The listing builds one solid part. Answer for the finished solid, in the listing's coordinates (mm). A direction names the side the tool comes from. Round coordinates to 2 decimals unless told otherwise and drop trailing zeros. Loops run counter-clockwise (first coordinate to the right, second up) from the corner with the lowest first, then second, coordinate; pieces in that order, holes last. Notation, with made-up numbers: (60.5, 21.25) -> (104.5, 21.25) arc R28 cw to (104.5, 47.25) -> close; hole circle Ø1 at (-18, 37). An arc over 180 degrees is marked (long way). Answer in a Markdown table with one row per item. Add a question column.
```python
from build123d import *

# Parameters (mm, degrees)
BOSS_EXTRUDE1_DEPTH = 1.524
CUT_EXTRUDE1_DEPTH  = 1.524
FILLET1_R           = 0.508
BOSS_EXTRUDE2_DEPTH = 6.223
BOSS_EXTRUDE3_START = -1.524
BOSS_EXTRUDE3_DEPTH = 1.524
CUT_EXTRUDE2_START  = -6.223
CUT_EXTRUDE2_DEPTH  = 6.223
FILLET2_R           = 0.254
SKETCH9_W           = 1.905
SKETCH9_H           = 23.876
CUT_EXTRUDE4_DEPTH  = 51.542276073
FILLET3_R           = 0.254


with BuildPart() as part:
    # Sketch2 → Boss-Extrude1 (new body)
    with BuildSketch(Plane(origin=(0, 0, 0), x_dir=(0, 0, -1), z_dir=(1, 0, 0))):
        with BuildLine():
            Line((-10.16, 10.851579944), (-10.16, 9.756379827))
            ThreePointArc((-10.16, 9.756379827), (-8.902698353, 7.16361824), (-6.088278228, 6.54534691))
            ThreePointArc((-6.088278228, 6.54534691), (-1.097578785, 7.201770952), (3.920718614, 6.808496661))
            ThreePointArc((3.920718614, 6.808496661), (7.044965017, 7.926917254), (7.619757818, 11.195157369))
            ThreePointArc((7.619757818, 11.195157369), (4.593793799, 26.843864795), (6.687175028, 42.644379261))
            ThreePointArc((6.687175028, 42.644379261), (5.465660141, 45.611386582), (2.312998216, 45.014767901))
            ThreePointArc((2.312998216, 45.014767901), (-6.944233805, 29.036045126), (-10.16, 10.851579944))
        make_face()
    extrude(amount=BOSS_EXTRUDE1_DEPTH)

    # Sketch3 → Cut-Extrude1 (cut)
    with BuildSketch(Plane(origin=(1.524, 0, 0), x_dir=(0, 0, -1), z_dir=(1, 0, 0))):
        with BuildLine():
            Line((-7.62, 10.851579944), (-7.62, 9.756379827))
            ThreePointArc((-7.62, 9.756379827), (-7.329853466, 9.15805023), (-6.680371899, 9.015372231))
            ThreePointArc((-6.680371899, 9.015372231), (-1.164335672, 9.74089354), (4.382203558, 9.306221955))
            ThreePointArc((4.382203558, 9.306221955), (5.103183497, 9.564319015), (5.23582799, 10.318528273))
            ThreePointArc((5.23582799, 10.318528273), (2.05490982, 26.768577734), (4.25548932, 43.378207999))
            ThreePointArc((4.25548932, 43.378207999), (-4.558282485, 28.164933022), (-7.62, 10.851579944))
        make_face()
    extrude(amount=-CUT_EXTRUDE1_DEPTH, mode=Mode.SUBTRACT)

    # Fillet1
    fillet1_edges = [part.edges().sort_by_distance(p)[0] for p in [
        (0.762, 43.378207999, -4.25548932),
    ]]
    fillet(fillet1_edges, radius=FILLET1_R)

    # Sketch4 → Boss-Extrude2 (add)
    with BuildSketch(Plane.ZY):
        with BuildLine():
            Line((8.89, 9.756379827), (8.89, 10.851579944))
            ThreePointArc((8.89, 10.851579944), (5.751258145, 28.600489074), (-3.284243768, 44.19648795))
            ThreePointArc((-3.284243768, 44.19648795), (-4.86057473, 44.49479729), (-5.471332174, 43.01129363))
            ThreePointArc((-5.471332174, 43.01129363), (-3.32435181, 26.806221264), (-6.427792904, 10.756842821))
            ThreePointArc((-6.427792904, 10.756842821), (-6.074074257, 8.745618135), (-4.151461086, 8.057359308))
            ThreePointArc((-4.151461086, 8.057359308), (1.130957229, 8.471332246), (6.384325063, 7.78035957))
            ThreePointArc((6.384325063, 7.78035957), (8.116275909, 8.160834235), (8.89, 9.756379827))
        make_face()
        with BuildLine():
            Line((7.62, 9.756379827), (7.62, 10.851579944))
            ThreePointArc((7.62, 10.851579944), (4.96917921, 26.995100943), (-2.704895567, 41.443239142))
            ThreePointArc((-2.704895567, 41.443239142), (-3.329273356, 41.593156599), (-3.601704042, 41.011689155))
            ThreePointArc((-3.601704042, 41.011689155), (-2.10574247, 25.541961828), (-5.23582799, 10.318528273))
            ThreePointArc((-5.23582799, 10.318528273), (-5.103183497, 9.564319015), (-4.382203558, 9.306221955))
            ThreePointArc((-4.382203558, 9.306221955), (1.164335672, 9.74089354), (6.680371899, 9.015372231))
            ThreePointArc((6.680371899, 9.015372231), (7.329853466, 9.15805023), (7.62, 9.756379827))
        make_face(mode=Mode.SUBTRACT)
    extrude(amount=BOSS_EXTRUDE2_DEPTH)

    # Sketch5 → Boss-Extrude3 (add)
    with BuildSketch(Plane(origin=(1.524, 0, 0), x_dir=(0, 0, -1), z_dir=(1, 0, 0)).offset(BOSS_EXTRUDE3_START)):
        with BuildLine():
            Line((7.009110806, 43.67080126), (6.148171078, 49.106560771))
            ThreePointArc((6.148171078, 49.106560771), (3.588810081, 46.474083877), (1.217761815, 43.67080126))
            Line((1.217761815, 43.67080126), (6.534669415, 42.12894069))
            ThreePointArc((6.534669415, 42.12894069), (6.765621389, 42.901799905), (7.009110806, 43.67080126))
        make_face()
    extrude(amount=BOSS_EXTRUDE3_DEPTH)

    # Sketch6 → Cut-Extrude2 (cut)
    with BuildSketch(Plane.ZY.offset(6.223).offset(CUT_EXTRUDE2_START)):
        with BuildLine():
            Line((8.89, 9.756379827), (8.89, 10.851579944))
            ThreePointArc((8.89, 10.851579944), (5.751258145, 28.600489074), (-3.284243768, 44.19648795))
            ThreePointArc((-3.284243768, 44.19648795), (-4.86057473, 44.49479729), (-5.471332174, 43.01129363))
            ThreePointArc((-5.471332174, 43.01129363), (-3.32435181, 26.806221264), (-6.427792904, 10.756842821))
            ThreePointArc((-6.427792904, 10.756842821), (-6.074074257, 8.745618135), (-4.151461086, 8.057359308))
            ThreePointArc((-4.151461086, 8.057359308), (1.130957229, 8.471332246), (6.384325063, 7.78035957))
            ThreePointArc((6.384325063, 7.78035957), (8.116275909, 8.160834235), (8.89, 9.756379827))
        make_face()
        with BuildLine():
            Line((8.8646, 9.756379827), (8.8646, 10.851579944))
            ThreePointArc((8.8646, 10.851579944), (5.727398631, 28.591777953), (-3.303668679, 44.180122351))
            ThreePointArc((-3.303668679, 44.180122351), (-4.848473022, 44.472465504), (-5.447015317, 43.018631917))
            ThreePointArc((-5.447015317, 43.018631917), (-3.29896297, 26.805468394), (-6.403953606, 10.74807653))
            ThreePointArc((-6.403953606, 10.74807653), (-6.054656442, 8.761992152), (-4.156075935, 8.082336561))
            ThreePointArc((-4.156075935, 8.082336561), (1.131624798, 8.496723472), (6.390246, 7.805059824))
            ThreePointArc((6.390246, 7.805059824), (8.100547461, 8.180778555), (8.8646, 9.756379827))
        make_face(mode=Mode.SUBTRACT)
    extrude(amount=CUT_EXTRUDE2_DEPTH, mode=Mode.SUBTRACT)

    # Fillet2
    fillet2_edges = [part.edges().sort_by_distance(p)[0] for p in [
        (0.762, 49.106560771, -6.148171078),
    ]]
    fillet(fillet2_edges, radius=FILLET2_R)

    # Sketch9 → Cut-Extrude4 (cut, through all)
    with BuildSketch(Plane.XY.offset(-1.27)):
        with Locations((-5.2705, 25.4)):
            Rectangle(SKETCH9_W, SKETCH9_H)
    extrude(amount=-CUT_EXTRUDE4_DEPTH, mode=Mode.SUBTRACT)

    # Fillet3
    fillet3_edges = [part.edges().sort_by_distance(p)[0] for p in [
        (1.524, 10.303979886, 10.16),
        (1.524, 31.419004876, 6.008417097),
        (1.524, 48.825128825, -6.053623792),
        (1.524, 7.16361824, 8.902698353),
        (1.524, 7.201770952, 1.097578785),
        (1.524, 7.926917254, -7.044965017),
        (1.524, 10.303979886, 7.62),
        (1.524, 9.15805023, 7.329853466),
        (1.524, 9.74089354, 1.164335672),
        (1.524, 9.564319015, -5.103183497),
        (1.524, 25.541961828, -2.10574247),
        (1.524, 27.381577524, -4.580766254),
        (1.524, 26.995100943, 4.96917921),
        (1.524, 41.593156599, -3.329273357),
        (1.524, 46.147271822, -6.616876402),
    ]]
    fillet(fillet3_edges, radius=FILLET3_R)


with BuildPart() as body_2:
    # Mirror2: mirrored copy
    add(part.part.mirror(Plane(origin=(-6.223, 10.851579944, -42.8625), x_dir=(0, 0, 1), z_dir=(-1, 0, 0))))


solid = body_2.part
```
Item 1: Flat-ended cylindrical pins translate along their axes: P1, Ø1, axis at y = 28, z = 8, coming from the +X side; P2, Ø0.9, axis at x = -11, y = 10.5, coming from the -Z side; P3, Ø1.5, axis at x = -11.5, z = -1.5, coming from the -Y side; P4, Ø0.5, axis at x = -9, y = 10, coming from the +Z side. Find the tip coordinate at first contact, or state that the pin passes through.
Item 2: Section B-B, the plane x = -10.25 is taken. Write down the section's boundary in (y, z) (1 decimal), and give its area (3 significant figures).
Item 3: Section A-A, the plane x = -7 is taken. Write down the section's boundary in (y, z) (1 decimal), and give its area (3 significant figures).
Item 4: For faces 4 (the flat face through (-7, 37.338, -3)), 5 (the cylindrical face through (-9.378, 28.353, 5.814)), 6 (the cylindrical face through (-10.02, 9.15, 7.32)), 7 (the flat face through (-6.223, 25, 6)), determine the directions among +Z, -Z, +X, -X, +Y, -Y from which every point of the face is accessible in a straight line to the end or side of a thin tool.
Item 5: The mould has two halves that part along Z. Classify faces 1 (the flat face through (-13, 10, 10.16)), 2 (the cylindrical face through (-9.38, 8.5, 1.06)), 3 (the cylindrical face through (-13.072, 7.19, 8.935)): +Z half, -Z half, draft (parallel to the pull), parting line (faces both ways), or undercut.
Item 6: Consider L1, parallel to Y at x = -11, z = 2; L2, parallel to Z at x = -11.25, y = 13; L3, parallel to Y at x = -8.25, z = 0. Determine where each line is inside the solid, lowest interval first. Write a range as from..to.
Here are the results:
| question | item | result |
|---|---|---|
| 1 | P1 | passes through |
| 1 | P2 | stops at z = -6.53 |
| 1 | P3 | stops at y = 8.36 |
| 1 | P4 | stops at z = 8.86 |
| 2 | outline | (7.8, 6.4) arc R25.4 cw to (8.1, -4.2) arc R2 ccw to (10.7, -6.4) arc R50.9 cw to (43, -5.4) arc R1.2 ccw to (44.2, -3.3) arc R51.7 ccw to (10.9, 8.9) -> (9.8, 8.9) arc R2 ccw to start; hole (9, 6.7) arc R26.7 cw to (9.3, -4.4) arc R0.8 ccw to (10.3, -5.2) arc R52.1 cw to (41, -3.6) arc R0.5 ccw to (41.4, -2.7) arc R50.5 ccw to (10.9, 7.6) -> (9.8, 7.6) arc R0.8 ccw to start |
| 2 | area | 111 mm² |
| 3 | outline | (7.8, 6.4) arc R25.4 cw to (8.1, -4.2) arc R2 ccw to (10.7, -6.4) arc R50.9 cw to (13.5, -5.5) -> (13.5, -4.2) arc R52.1 ccw to (10.3, -5.2) arc R0.8 cw to (9.3, -4.4) arc R26.7 ccw to (9, 6.7) arc R0.8 cw to (9.8, 7.6) -> (10.9, 7.6) arc R50.5 cw to (41.4, -2.7) arc R0.5 cw to (41, -3.6) arc R52.1 ccw to (37.3, -2.8) -> (37.3, -4.1) arc R50.9 cw to (43, -5.4) arc R1.2 ccw to (44.2, -3.3) arc R51.7 ccw to (10.9, 8.9) -> (9.8, 8.9) arc R2 ccw to start |
| 3 | area | 80.6 mm² |
| 4 | face 4 | -Z, +X |
| 4 | face 5 | +Z, +X, +Y |
| 4 | face 6 | +X, -X |
| 4 | face 7 | +Z, -Z, +X, +Y, -Y |
| 5 | face 1 | +Z half |
| 5 | face 2 | undercut |
| 5 | face 3 | parting line |
| 6 | L1 | y = 8.46..9.71, 34..36.6 |
| 6 | L2 | z = -5.64..-4.33, 7.57..8.82 |
| 6 | L3 | y = 8.5..9.75, 37.52..39.81 |
